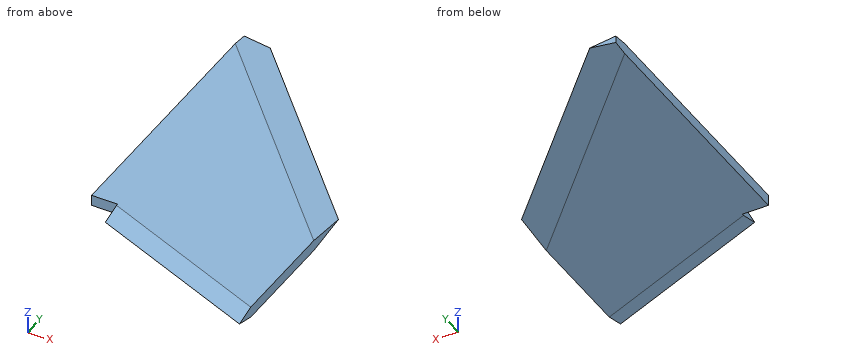
from build123d import *

# Parameters (mm, degrees)
SKETCH2_W                = 11.43
SKETCH2_H                = 117.475
BOSS_EXTRUDE3_DEPTH      = 4.7498
CUT_EXTRUDE17_DEPTH      = 5.08
CUT_EXTRUDE17_DEPTH_BACK = 101.6
CUT_EXTRUDE18_DEPTH      = 101.6
CUT_EXTRUDE18_DEPTH_BACK = 127


with BuildPart() as part:
    # Sketch2 → Boss-Extrude3 (new body)
    with BuildSketch(Plane.XY):
        Polygon((76.2, -30.9118), (0, 0), (0, 127), (76.2, 45.2882), align=None)
        with Locations((-5.715, 68.2625)):
            Rectangle(SKETCH2_W, SKETCH2_H)
    extrude(amount=BOSS_EXTRUDE3_DEPTH)

    # Sketch8 → Cut-Extrude17 (cut, two sides: drawn at the far end of the back side and taken through both)
    with BuildSketch(Plane(origin=(0, 0, 0), x_dir=(0, 0, -1), z_dir=(-0.9266549506898317, 0.37591302499650847, 0)).offset(-CUT_EXTRUDE17_DEPTH_BACK)):
        Polygon((-2.3749, 0), (3e-09, -8.038518146), (0.750296228, -8.038518146), (0.750296228, 2.310233708), (-5.314343575, 2.310233708), (-5.314343575, -8.038518146), (-4.749800003, -8.038518146), align=None)
    extrude(amount=CUT_EXTRUDE17_DEPTH + CUT_EXTRUDE17_DEPTH_BACK, mode=Mode.SUBTRACT)

    # Sketch9 → Cut-Extrude18 (cut, two sides: drawn at the far end of the back side and taken through both)
    with BuildSketch(Plane(origin=(12.854537069, -13.784348584, 0), x_dir=(0, 0, -1), z_dir=(0.6820103942193665, -0.731342479401234, 0)).offset(-CUT_EXTRUDE18_DEPTH_BACK)):
        Polygon((-2.3749, 86.615320066), (0, 73.622586943), (0.872559858, 73.622586943), (0.872559858, 91.301528403), (-6.531219552, 91.301528403), (-6.531219552, 73.622586943), (-4.7498, 73.622586943), align=None)
    extrude(amount=CUT_EXTRUDE18_DEPTH + CUT_EXTRUDE18_DEPTH_BACK, mode=Mode.SUBTRACT)


solid = part.part
Design review of the part built by this model. Coordinates are the model's own, in mm. Round coordinates to 2 decimals unless told otherwise and drop trailing zeros. Write each loop counter-clockwise with the first axis right and the second up, starting at its lowest first coordinate (ties: lowest second). Pieces come first, ordered by that corner, then holes.
Item 1: For pin 1 Ø2.5 at (y, z) = (6.5, 3) entering from -X, flat-tipped, find the tip position at first contact; note if it passes through.
Item 2: Consider section D-D on x = 44.5. Give the boundary of the cut face in (y, z).
Item 3: Consider section A-A on y = 91. Give the boundary of the cut face in (x, z), and give its area (3 significant figures).
Item 4: Consider section B-B on x = 11.5. Give the boundary of the cut face in (y, z).
Item 5: Wall thickness on L1, parallel to Z at x = 10, y = 107; L2, parallel to Z at x = 61.5, y = -17: over which ranges is each line inside the solid? List them lowest first.
Item 6: Consider section C-C on y = -5.5. Give the boundary of the cut face in (x, z), and give its area (3 significant figures).
Check values:
1. pin 1: stops at x = 0
2. outline: (-18.05, 2.37) - (-9.38, 0) - (60.23, 0) - (79.28, 2.37) - (60.23, 4.75) - (-9.38, 4.75) - close
3. outline: (-11.43, 0) - (15.81, 0) - (33.57, 2.37) - (15.81, 4.75) - (-11.43, 4.75) - close
3. area: 172 mm2
4. outline: (-4.67, 2.37) - (4.01, 0) - (95.62, 0) - (114.67, 2.37) - (95.62, 4.75) - (4.01, 4.75) - close
5. L1: z = 1.22 to 3.53
5. L2: z = 0.2 to 4.55
6. outline: (13.56, 2.37) - (34.94, 0) - (76.2, 0) - (76.2, 4.75) - (34.94, 4.75) - close
6. area: 247 mm2
